Build history of the part. All positions in model axes, mm. Face numbers are marked on the shaded views. A direction names the side the tool comes from. Coordinates: 2 decimals unless noted, no trailing zeros. Order: outer loops, then holes, each group sorted by start corner. A loop starts at its lowest first (then second) coordinate and runs counter-clockwise, first axis right, second up. Notation, with made-up numbers: (10, -15) - (65, -15) arc R19 cw to (65, -9) - close; hole circle Ø9 at (33.5, 61). An arc over 180 degrees is marked (long way). One line per item, written item: value.
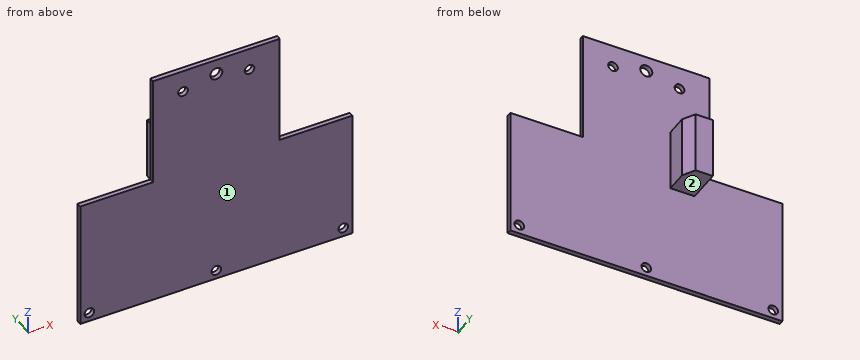
from build123d import *

# Parameters (mm, degrees)
SKETCH_1_R      = 1.6
SKETCH_1_R_2    = 2
EXTRUDE_1_DEPTH = 1.54
SKETCH_2_W      = 8
SKETCH_2_H      = 20.5
EXTRUDE_2_DEPTH = 11
CHAMFER_1_SIZE  = 4
CHAMFER_1_SIZE2 = 2.309401077


with BuildPart() as part:
    # Эскиз1 → Бобышка-Вытянуть1 (new body)
    with BuildSketch(Plane(origin=(0, 0, 0), x_dir=(1, 0, 0), z_dir=(0, 1, 0))):
        Polygon((-21, 0), (21, 0), (21, 37), (45, 37), (45, 80), (-45, 80), (-45, 37), (-21, 37), align=None)
        with Locations(Location((11, 7.5, 0), (0, 0, 270))):
            Circle(SKETCH_1_R, mode=Mode.SUBTRACT)
        with Locations(Location((42, 77, 0), (0, 0, 270))):
            Circle(SKETCH_1_R, mode=Mode.SUBTRACT)
        with Locations(Location((0, 77, 0), (0, 0, 270))):
            Circle(SKETCH_1_R, mode=Mode.SUBTRACT)
        with Locations(Location((0, 5, 0), (0, 0, 270))):
            Circle(SKETCH_1_R_2, mode=Mode.SUBTRACT)
        with Locations(Location((-42, 77, 0), (0, 0, 90))):
            Circle(SKETCH_1_R, mode=Mode.SUBTRACT)
        with Locations(Location((-11, 7.5, 0), (0, 0, 90))):
            Circle(SKETCH_1_R, mode=Mode.SUBTRACT)
    extrude(amount=EXTRUDE_1_DEPTH)

    # Эскиз2 → Бобышка-Вытянуть2 (add)
    with BuildSketch(Plane(origin=(0, 1.54, 0), x_dir=(1, 0, 0), z_dir=(0, 1, 0))):
        with Locations((-12, 34.75)):
            Rectangle(SKETCH_2_W, SKETCH_2_H)
    extrude(amount=EXTRUDE_2_DEPTH)

    # Фаска1
    chamfer_1_edges = [part.edges().sort_by_distance(p)[0] for p in [
        (-8, 12.54, -34.75),
    ]]
    chamfer_1_side = [part.faces().sort_by_distance(p)[0] for p in [
        (-8, 7.04, -34.75),
    ]]
    chamfer(chamfer_1_edges, length=CHAMFER_1_SIZE, length2=CHAMFER_1_SIZE2, reference=chamfer_1_side[0])


solid = part.part
1. Band-saw the part on B-B, the plane z = -29. Give the cut face in (x, y), and give its area (3 significant figures).
Values found:
outline: (-21, 0) - (21, 0) - (21, 1.54) - (-8, 1.54) - (-8, 8.54) - (-10.31, 12.54) - (-16, 12.54) - (-16, 1.54) - (-21, 1.54) - close
area: 148 mm2
2. 3-axis set-ups, long thin cutter, end or side, ignore diameter. For the marked faces 1 and 2: which of +Z, -Z, +X, -X, +Y, -Y reach the whole face in a straight line?
Values found:
face 1: +Z, -Z, +X, -X, -Y
face 2: -Z, +X, -X, +Y
3. Band-saw the part on A-A, the plane x = -42. Give the cut face in (y, z), and give its area (3 significant figures).
Values found:
outline: (0, -80) - (1.54, -80) - (1.54, -78.6) - (0, -78.6) - close; (0, -75.4) - (1.54, -75.4) - (1.54, -37) - (0, -37) - close
area: 61.3 mm2
4. Flat gauge pins, fed straight in: P1, Ø4, axis at x = 42, z = -77, coming from the +Y side; P2, Ø5.5, axis at y = 6, z = -31, coming from the -X side; P3, Ø1.9, axis at x = 11, z = -7.5, coming from the +Y side; P4, Ø0.5, axis at x = 29, y = 1, coming from the +Z side. Where does each tip first touch, or does it go through?
Values found:
P1: stops at y = 1.54
P2: stops at x = -16
P3: passes through
P4: stops at z = -37
5. Probe line 1 along X through (y, z) = (1, -7.5); line 2 along X through (y, z) = (1.25, -77); line 3 along X through (y, z) = (0.9, -5). List the from-to ranges inside material, lowest first.
Values found:
line 1: x = -21 to -12.6, -9.4 to 9.4, 12.6 to 21
line 2: x = -45 to -43.6, -40.4 to -1.6, 1.6 to 40.4, 43.6 to 45
line 3: x = -21 to -2, 2 to 21
6. Band-saw the part on C-C, the plane x = -14. Give the cut face in (y, z), and give its area (3 significant figures).
Values found:
outline: (0, -80) - (1.54, -80) - (1.54, -45) - (12.54, -45) - (12.54, -24.5) - (1.54, -24.5) - (1.54, 0) - (0, 0) - close
area: 349 mm2
7. Band-saw the part on D-D, the plane x = 11. Give the cut face in (y, z), and give its area (3 significant figures).
Values found:
outline: (0, -80) - (1.54, -80) - (1.54, -9.1) - (0, -9.1) - close; (0, -5.9) - (1.54, -5.9) - (1.54, 0) - (0, 0) - close
area: 118 mm2
